Can you work these out from the model? Positions are in its coordinate system, mm. Face numbers are marked on the shaded views. A direction names the side the tool comes from. Coordinates: 2 decimals unless noted, no trailing zeros. Order: outer loops, then holes, each group sorted by start corner. A loop starts at its lowest first (then second) coordinate and runs counter-clockwise, first axis right, second up. Notation, with made-up numbers: M -29,75.5 L 12,75.5 A17 ccw 12,105.5 Z; hole C -13.5,73 d1. An arc over 180 degrees is marked long. Answer as a JSON object with one key per item and string values.
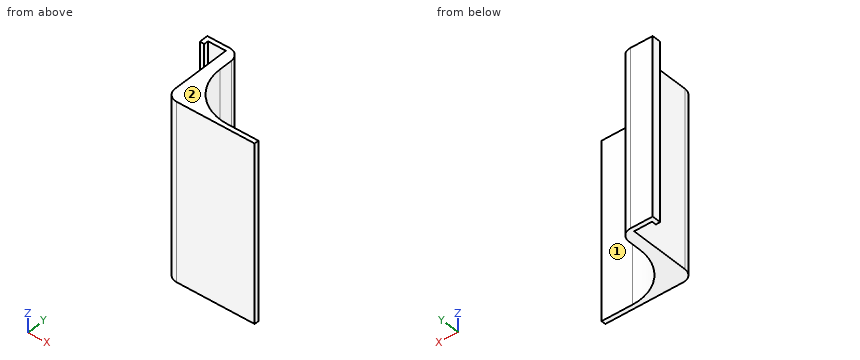
from build123d import *

# Parameters (mm, degrees)
SKETCH1_W           = 40
SKETCH1_H           = 80
BOSS_EXTRUDE4_DEPTH = 2
SKETCH4_W           = 5
SKETCH4_H           = 80
BOSS_EXTRUDE5_DEPTH = 32
FILLET3_R           = 21
SKETCH5_W           = 80
SKETCH5_H           = 2
BOSS_EXTRUDE6_DEPTH = 10
SKETCH6_W           = 2
SKETCH6_H           = 80
BOSS_EXTRUDE7_DEPTH = 2
FILLET4_R           = 5


with BuildPart() as part:
    # Sketch1 → Boss-Extrude4 (new body)
    with BuildSketch(Plane(origin=(0, 0, 0), x_dir=(1, 0, 0), z_dir=(0, 1, 0))):
        Rectangle(SKETCH1_W, SKETCH1_H)
    extrude(amount=BOSS_EXTRUDE4_DEPTH)

    # Sketch4 → Boss-Extrude5 (add)
    with BuildSketch(Plane(origin=(0, 2, 0), x_dir=(1, 0, 0), z_dir=(0, 1, 0))):
        with Locations((-17.5, 0)):
            Rectangle(SKETCH4_W, SKETCH4_H)
    extrude(amount=BOSS_EXTRUDE5_DEPTH)

    # Fillet3
    fillet3_edges = [part.edges().sort_by_distance(p)[0] for p in [
        (-15, 2, 0),
    ]]
    fillet(fillet3_edges, radius=FILLET3_R)

    # Sketch5 → Boss-Extrude6 (add)
    with BuildSketch(Plane.ZY.offset(20)):
        with Locations((0, 33)):
            Rectangle(SKETCH5_W, SKETCH5_H)
    extrude(amount=BOSS_EXTRUDE6_DEPTH)

    # Sketch6 → Boss-Extrude7 (add)
    with BuildSketch(Plane.XZ.offset(-32)):
        with Locations((-29, 0)):
            Rectangle(SKETCH6_W, SKETCH6_H)
    extrude(amount=BOSS_EXTRUDE7_DEPTH)

    # Fillet4
    fillet4_edges = [part.edges().sort_by_distance(p)[0] for p in [
        (-15, 34, 0),
        (-20, 0, 0),
    ]]
    fillet(fillet4_edges, radius=FILLET4_R)


solid = part.part
Item 1: Which directions (+Z, -Z, +X, -X, +Y, -Y) give clear straight access to the entire face, cutting with the end or side of a thin tool? Please do the marked faces 1 and 2.
Answers follow:
{"face 1": "+Z, -Z, +X, +Y", "face 2": "+Z, +X, -X, +Y, -Y"}
Item 2: I'm going to push flat-ended pins straight in: pin 1 (6.5 mm diameter, centred on x = -22.5, z = -4, fed in from -Y); pin 2 (2 mm diameter, centred on y = 31.5, z = 10, fed in from +X); pin 3 (3 mm diameter, centred on y = 24.5, z = -7, fed in from +X). Where does each tip first touch, or does it pass through?
Answers follow:
{"pin 1": "stops at y = 2.37", "pin 2": "stops at x = -15.23", "pin 3": "stops at x = -15"}
Item 3: Please list where these lines run through material, in increasing order: line 1 (Y direction, x = 7, z = -20); line 2 (X direction, y = 24, z = 15.5); line 3 (X direction, y = 31.5, z = -6.5).
Answers follow:
{"line 1": "y = 0 to 2", "line 2": "x = -20 to -15", "line 3": "x = -30 to -28, -20 to -15.67"}
Item 4: I want a section at A-A, the plane y = 31. Write out the boundary of the cut face in (x, z), plus the area to 3 significant figures.
Answers follow:
{"outline": "M -30,-40 L -28,-40 L -28,40 L -30,40 Z; M -20,-40 L -15.42,-40 L -15.42,40 L -20,40 Z", "area": "527 mm^2"}
Item 5: I want a section at B-B, the plane z = 27. Write out the boundary of the cut face in (x, y).
Answers follow:
{"outline": "M -30,30 L -28,30 L -28,32 L -20,32 L -20,5 A5 ccw -15,0 L 20,0 L 20,2 L 6,2 A21 cw -15,23 L -15,29 A5 ccw -20,34 L -30,34 Z"}
Item 6: I want a section at D-D, the plane y = 19.5. Write out the boundary of the cut face in (x, z).
Answers follow:
{"outline": "M -20,-40 L -14.71,-40 L -14.71,40 L -20,40 Z"}
Item 7: I want a section at C-C, the plane x = 12. Write out the boundary of the cut face in (y, z), plus the area to 3 significant figures.
Answers follow:
{"outline": "M 0,-40 L 2,-40 L 2,40 L 0,40 Z", "area": "160 mm^2"}
